```python
from build123d import *

# Parameters (mm, degrees)
SKETCH1_W                                     = 127
SKETCH1_H                                     = 76.2
BOSS_EXTRUDE1_DEPTH                           = 6.35
SKETCH3_R                                     = 1.5367
SKETCH3_W                                     = 4.6228
SKETCH3_H                                     = 4.6228
BOSS_EXTRUDE2_DEPTH                           = 6.35
CBORE_FOR_8_BUTTON_HEAD_CAP_SCREW1_AT_2_COUNT = 2
CBORE_FOR_8_BUTTON_HEAD_CAP_SCREW1_AT_2_PITCH = 57.667566167
CBORE_FOR_8_BUTTON_HEAD_CAP_SCREW1_AT_3_COUNT = 2
CBORE_FOR_8_BUTTON_HEAD_CAP_SCREW1_AT_3_PITCH = 60.644913617
SKETCH4_R                                     = 1.6
CUT_EXTRUDE1_DEPTH                            = 185.758568144


with BuildPart() as part:
    # Sketch1 → Boss-Extrude1 (new body)
    with BuildSketch(Plane(origin=(0, 0, 0), x_dir=(1, 0, 0), z_dir=(0, 1, 0))):
        with Locations((63.5, 38.1)):
            Rectangle(SKETCH1_W, SKETCH1_H)
    extrude(amount=BOSS_EXTRUDE1_DEPTH)

    # Sketch3 → Boss-Extrude2 (add)
    with BuildSketch(Plane(origin=(104.775, 0, 0), x_dir=(0, 0, -1), z_dir=(1, 0, 0))):
        Polygon((0, 6.35), (-0.3556, 89.7636), (99.7458, 83.9978), (99.7458, 6.35), align=None)
        with Locations((86.986368363, 50.326031637)):
            Circle(SKETCH3_R, mode=Mode.SUBTRACT)
        with Locations((86.986368363, 32.596831637)):
            Circle(SKETCH3_R, mode=Mode.SUBTRACT)
        with Locations((8.3058, 55.7022)):
            Rectangle(SKETCH3_W, SKETCH3_H, mode=Mode.SUBTRACT)
        with Locations((8.3058, 68.4022)):
            Rectangle(SKETCH3_W, SKETCH3_H, mode=Mode.SUBTRACT)
        with Locations((35.246568363, 41.461431637)):
            Rectangle(SKETCH3_W, SKETCH3_H, mode=Mode.SUBTRACT)
        with Locations((78.3844, 75.3364)):
            Rectangle(SKETCH3_W, SKETCH3_H, mode=Mode.SUBTRACT)
        with Locations((8.3058, 81.1022)):
            Rectangle(SKETCH3_W, SKETCH3_H, mode=Mode.SUBTRACT)
        with Locations((35.246568363, 54.161431637)):
            Rectangle(SKETCH3_W, SKETCH3_H, mode=Mode.SUBTRACT)
        with Locations((35.246568363, 28.761431637)):
            Rectangle(SKETCH3_W, SKETCH3_H, mode=Mode.SUBTRACT)
        with Locations((65.6844, 75.3364)):
            Rectangle(SKETCH3_W, SKETCH3_H, mode=Mode.SUBTRACT)
        with Locations((52.9844, 75.3364)):
            Rectangle(SKETCH3_W, SKETCH3_H, mode=Mode.SUBTRACT)
    boss_extrude2 = extrude(amount=BOSS_EXTRUDE2_DEPTH)

    # Sketch6 → CBORE for #8 Button Head Cap Screw1 (revolve, cut)
    with BuildSketch(Plane(origin=(104.775, 75.3364, -65.6844), x_dir=(0, 0, 1), z_dir=(0, 1, 0))):
        Polygon((0, 0), (0, 22.225), (2.2479, 22.225), (2.2479, 2.7178), (4.36626, 2.7178), (4.36626, 0), align=None)
    cbore_for_8_button_head_cap_screw1 = revolve(axis=Axis((98.425, 75.3364, -65.6844), (1, 0, 0)), mode=Mode.SUBTRACT)

    # CBORE for #8 Button Head Cap Screw1 at 2: CBORE for #8 Button Head Cap Screw1 ×2
    with Locations(*[Vector(0, 0.09998341153022382, 0.9949891041708838) * (i * CBORE_FOR_8_BUTTON_HEAD_CAP_SCREW1_AT_2_PITCH) for i in range(1, CBORE_FOR_8_BUTTON_HEAD_CAP_SCREW1_AT_2_COUNT)]):
        add(cbore_for_8_button_head_cap_screw1, mode=Mode.SUBTRACT)

    # CBORE for #8 Button Head Cap Screw1 at 3: CBORE for #8 Button Head Cap Screw1 ×2
    with Locations(*[Vector(0, -0.32375674774697566, 0.9461403533769719) * (i * CBORE_FOR_8_BUTTON_HEAD_CAP_SCREW1_AT_3_PITCH) for i in range(1, CBORE_FOR_8_BUTTON_HEAD_CAP_SCREW1_AT_3_COUNT)]):
        add(cbore_for_8_button_head_cap_screw1, mode=Mode.SUBTRACT)

    # Mirror1: Boss-Extrude2, CBORE for #8 Button Head Cap Screw1 across plane
    add(boss_extrude2.mirror(Plane(origin=(63.5, 0, 0), x_dir=(0, 0, 1), z_dir=(1, 0, 0))))
    add(cbore_for_8_button_head_cap_screw1.mirror(Plane(origin=(63.5, 0, 0), x_dir=(0, 0, 1), z_dir=(1, 0, 0))), mode=Mode.SUBTRACT)

    # Mirror1 copy 1 sketch → Mirror1 copy 1 (revolve, cut)
    with BuildSketch(Plane(origin=(22.225, 81.1022, -8.3058), x_dir=(0, 0, 1), z_dir=(0, 1, 0))):
        Polygon((0, 0), (0, -22.225), (2.2479, -22.225), (2.2479, -2.7178), (4.36626, -2.7178), (4.36626, 0), align=None)
    revolve(axis=Axis((28.575, 81.1022, -8.3058), (1, 0, 0)), mode=Mode.SUBTRACT)

    # Mirror1 copy 2 sketch → Mirror1 copy 2 (revolve, cut)
    with BuildSketch(Plane(origin=(22.225, 55.7022, -8.3058), x_dir=(0, 0, 1), z_dir=(0, 1, 0))):
        Polygon((0, 0), (0, -22.225), (2.2479, -22.225), (2.2479, -2.7178), (4.36626, -2.7178), (4.36626, 0), align=None)
    revolve(axis=Axis((28.575, 55.7022, -8.3058), (1, 0, 0)), mode=Mode.SUBTRACT)

    # Sketch4 → Cut-Extrude1 (cut, through all)
    with BuildSketch(Plane.XZ):
        with Locations(Location((76.999706662, -26.448823052, 0), (0, 0, 270))):
            Circle(SKETCH4_R)
        with Locations(Location((47.000293338, -26.448823052, 0), (0, 0, 270))):
            Circle(SKETCH4_R)
        with Locations(Location((81.99934001, -58.48420412, 0), (0, 0, 270))):
            Circle(SKETCH4_R)
        with Locations(Location((42.00065999, -58.48420412, 0), (0, 0, 270))):
            Circle(SKETCH4_R)
    extrude(amount=-CUT_EXTRUDE1_DEPTH, mode=Mode.SUBTRACT)


solid = part.part
```
Geometry check sheet. Reference: the model listing, model coordinates, mm. A direction names the side the tool comes from. Round coordinates to 2 decimals unless told otherwise and drop trailing zeros. Order: outer loops, then holes, each group sorted by start corner. A loop starts at its lowest first (then second) coordinate and runs counter-clockwise, first axis right, second up. Notation, with made-up numbers: (36.5, -24.5) -> (45.5, -24.5) arc R26 ccw to (45.5, 0.5) -> close; hole circle Ø6 at (-22, -33). An arc over 180 degrees is marked (long way). Return JSON: item names as keys, results as strings. Group by question number.
Q1. Section check A-A, the plane z = -87. Record the boundary of the cut face in (x, y) (3 decimals).
Q2. Section check B-B, the plane y = 29. Record the boundary of the cut face in (x, z) (3 decimals).
Q3. Release check for a two-part mould opening along Z. For faces 6 (the flat face through (107.493, 75, -69)), 7 (the cylindrical face through (19.09, 49.39, -85.77)), 8 (the flat face through (63, 6.35, -39)) record: released by +Z, released by -Z, zero draft, split by the parting line, or undercut.
Q4. Material ranges on probe 1 along X at (y, z) = (44.5, -27.5) (3 decimals); probe 2 along Y at (x, z) = (43.5, -20); probe 3 along X at (y, z) = (73, -68.5) (3 decimals), recorded low to high. Write a range as from..to.
Q5. Section check D-D, the plane z = -7.5. Count the separate pieces of the cut face and the enclosed holes in it, plus the area to 3 significant figures.
Q6. Section check C-C, the plane x = 52.5. Record the boundary of the cut face in (y, z).
Q7. Tool access check on faces 1 (the flat face through (119, 6.35, -39)), 2 (the flat face through (19.507, 81, -11)), 3 (the flat face through (63, 0, -39)), 4 (the flat face through (108, 75, -80.696)), 5 (the flat face through (8, 6.35, -39)). Record the directions out of +Z, -Z, +X, -X, +Y, -Y that give a thin tool (end or side, any length) a straight path to the whole face; none if there is none.
Q8. Gauge pin test, flat ends, axial feed: pin 1 (12 mm diameter, centred on x = 89.5, y = 9.5, fed in from -Z); pin 2 (1 mm diameter, centred on y = 78.5, z = -45, fed in from -X) (3 decimals); pin 3 (3 mm diameter, centred on x = 109.5, z = -65.5, fed in from +Y). Record the tip position at first contact, or that the pin passes through.
Numbers:
{
 "1": {"outline": "(15.875, 6.35) -> (22.225, 6.35) -> (22.225, 31.06) -> (15.875, 31.06) -> close; (15.875, 34.133) -> (22.225, 34.133) -> (22.225, 48.789) -> (15.875, 48.789) -> close; (15.875, 51.863) -> (22.225, 51.863) -> (22.225, 84.732) -> (15.875, 84.732) -> close; (104.775, 6.35) -> (111.125, 6.35) -> (111.125, 31.06) -> (104.775, 31.06) -> close; (104.775, 34.133) -> (111.125, 34.133) -> (111.125, 48.789) -> (104.775, 48.789) -> close; (104.775, 51.863) -> (111.125, 51.863) -> (111.125, 84.732) -> (104.775, 84.732) -> close"},
 "2": {"outline": "(15.875, -99.746) -> (22.225, -99.746) -> (22.225, -37.558) -> (15.875, -37.558) -> close; (15.875, -32.935) -> (22.225, -32.935) -> (22.225, 0.097) -> (15.875, 0.097) -> close; (104.775, -99.746) -> (111.125, -99.746) -> (111.125, -37.558) -> (104.775, -37.558) -> close; (104.775, -32.935) -> (111.125, -32.935) -> (111.125, 0.097) -> (104.775, 0.097) -> close"},
 "3": {"face 6": "undercut", "face 7": "undercut", "face 8": "zero draft"},
 "4": {"probe 1": "15.875..22.225, 104.775..111.125", "probe 2": "0..6.35", "probe 3": "15.875..19.507, 107.493..111.125"},
 "5": {"separate pieces": "7", "enclosed holes": "0", "area": "1,640 mm^2"},
 "6": {"outline": "(0, -76.2) -> (6.35, -76.2) -> (6.35, 0) -> (0, 0) -> close"},
 "7": {"face 1": "+Z, -Z, +X, +Y", "face 2": "none", "face 3": "+Z, -Z, +X, -X, -Y", "face 4": "+X, -X", "face 5": "+Z, -Z, -X, +Y"},
 "8": {"pin 1": "z = -76.2", "pin 2": "x = 15.875", "pin 3": "y = 86.06"}
}
